```python
from build123d import *

# Parameters (mm, degrees)
F1_DEPTH = 50
F3_DEPTH = 25


with BuildPart() as f1:
    # F0 (on Top) → F1 (new body)
    with BuildSketch(Plane.XY):
        with BuildLine():
            ThreePointArc((0, 0), (25, 7.583426), (50, 0))
            Line((50, 0), (50, 0.6))
            ThreePointArc((50, 0.6), (25, 8.183426), (0, 0.6))
            Line((0, 0.6), (0, 0))
        make_face()
    extrude(amount=F1_DEPTH)

    # F2 (on Front) → F3 (cut)
    with BuildSketch(Plane.XZ):
        Polygon((25, 35), (18, 20), (32, 20), align=None)
    extrude(amount=-F3_DEPTH, mode=Mode.SUBTRACT)


solid = f1.part
```
For this review, take the finished solid that the model builds, in its own axes (mm). Give positions to 0.01 mm unless a question says otherwise; leave off trailing zeros. Order: outer loops, then holes, each group sorted by start corner. A loop starts at its lowest first (then second) coordinate and runs counter-clockwise, first axis right, second up.
1) Take a section at A-A (x = 26.5). Give the boundary of the cut face in (y, z).
2) Take a section at D-D (x = 5). Give the boundary of the cut face in (y, z).
3) Take a section at C-C (z = 39.5). Give the boundary of the cut face in (x, y).
4) Insertion check: pin 1 (1.5 mm diameter, centred on y = 3.5, z = 37.5, fed in from -X); pin 2 (6 mm diameter, centred on x = 40.5, z = 35.5, fed in from +Y); pin 3 (1 mm diameter, centred on x = 21, y = 6, fed in from -Z); pin 4 (5 mm diameter, centred on x = 12, z = 7, fed in from -Y). Each pin has a flat end and moves straight along its axis. Give the tip position at first contact, or say it passes through.
5) Wall thickness on line 1 (X direction, y = 0.75, z = 30); line 2 (X direction, y = 1.5, z = 4.5); line 3 (Z direction, x = 30, y = 7.5): over which ranges is each line inside the solid? List them lowest first.
6) Take a section at B-B (y = 3.5). Give the boundary of the cut face in (x, z).
Derived:
1. outline: (7.56, 0) - (8.16, 0) - (8.16, 20) - (7.56, 20) - close; (7.56, 31.79) - (8.16, 31.79) - (8.16, 50) - (7.56, 50) - close
2. outline: (2.89, 0) - (3.49, 0) - (3.49, 50) - (2.89, 50) - close
3. outline: (0, 0) arc R45 cw to (50, 0) - (50, 0.6) arc R45 ccw to (0, 0.6) - close
4. pin 1: stops at x = 3.56
4. pin 2: stops at y = 6.41
4. pin 3: passes through
4. pin 4: stops at y = 4.83
5. line 1: x = 0.23 to 1.16, 48.84 to 49.77
5. line 2: x = 1.4 to 2.41, 47.59 to 48.6
5. line 3: z = 0 to 20, 24.29 to 50
6. outline: (5.01, 0) - (6.27, 0) - (6.27, 50) - (5.01, 50) - close; (43.73, 0) - (44.99, 0) - (44.99, 50) - (43.73, 50) - close
